from build123d import *

# Parameters (mm, degrees)
SKETCH1_R      = 2.35
EXTRUDE1_DEPTH = 3.1


with BuildPart() as part:
    # Sketch1 → Extrude1 (new body)
    with BuildSketch(Plane.XY):
        Polygon((-33.263157114, 29.408489293), (-41.013157114, 29.408489293), (-41.013157114, 12.158489293), (-33.263157114, 12.158489293), (-33.263157114, 9.058489293), (-18.263157114, 9.058489293), (-18.263157114, 12.158489293), (-10.513157114, 12.158489293), (-10.513157114, 29.408489293), (-18.263157114, 29.408489293), (-18.263157114, 32.508489293), (-33.263157114, 32.508489293), align=None)
        with Locations(Location((-14.388157114, 26.058489293, 0), (0, 0, 180))):
            Circle(SKETCH1_R, mode=Mode.SUBTRACT)
        with Locations(Location((-37.138157114, 26.058489293, 0), (0, 0, 180))):
            Circle(SKETCH1_R, mode=Mode.SUBTRACT)
        with Locations(Location((-25.763157114, 15.508489293, 0), (0, 0, 180))):
            Circle(SKETCH1_R, mode=Mode.SUBTRACT)
        with BuildLine():
            Line((-37.138157114, 21.287155622), (-37.138157114, 14.158489293))
            ThreePointArc((-37.138157114, 14.158489293), (-36.845263895, 13.451382512), (-36.138157114, 13.158489293))
            Line((-36.138157114, 13.158489293), (-33.725119975, 13.158489293))
            ThreePointArc((-33.725119975, 13.158489293), (-33.328320215, 13.240584097), (-32.996670851, 13.473389392))
            Line((-32.996670851, 13.473389392), (-28.585897467, 18.16325141))
            ThreePointArc((-28.585897467, 18.16325141), (-25.763157114, 19.383489293), (-22.940416761, 18.16325141))
            Line((-22.940416761, 18.16325141), (-18.529643377, 13.473389392))
            ThreePointArc((-18.529643377, 13.473389392), (-18.197994013, 13.240584097), (-17.801194253, 13.158489293))
            Line((-17.801194253, 13.158489293), (-15.388157114, 13.158489293))
            ThreePointArc((-15.388157114, 13.158489293), (-14.681050333, 13.451382512), (-14.388157114, 14.158489293))
            Line((-14.388157114, 14.158489293), (-14.388157114, 21.287155622))
            ThreePointArc((-14.388157114, 21.287155622), (-14.611907088, 21.917580794), (-15.183028909, 22.265890734))
            ThreePointArc((-15.183028909, 22.265890734), (-17.128195891, 23.318450516), (-18.180755673, 25.263617499))
            ThreePointArc((-18.180755673, 25.263617499), (-18.529065613, 25.834739319), (-19.159490785, 26.058489293))
            Line((-19.159490785, 26.058489293), (-32.366823443, 26.058489293))
            ThreePointArc((-32.366823443, 26.058489293), (-32.997248615, 25.834739319), (-33.345558555, 25.263617499))
            ThreePointArc((-33.345558555, 25.263617499), (-34.398118337, 23.318450516), (-36.343285319, 22.265890734))
            ThreePointArc((-36.343285319, 22.265890734), (-36.91440714, 21.917580794), (-37.138157114, 21.287155622))
        make_face(mode=Mode.SUBTRACT)
    extrude(amount=EXTRUDE1_DEPTH)


solid = part.part
Here's how the part is built. I have some questions about the finished solid (model axes, mm). A direction names the side the tool comes from. Coordinates: 2 decimals unless noted, no trailing zeros. Loops run counter-clockwise (first coordinate to the right, second up) from the corner with the lowest first, then second, coordinate; pieces in that order, holes last.
1. If we mould it in two halves opening along Y, with no side actions, what happens to faces 1 (the flat face through (-37, 12.158, 2)), 2 (the flat face through (-33.263, 11, 2)), 3 (the flat face through (-17, 13.158, 2))? For each: pulls with the +Y half, pulls with the -Y half, needs draft (parallel to the pull), parting line crosses it, or undercut.
2. I need wall thicknesses on L1, parallel to X at y = 18, z = 0.25; L2, parallel to X at y = 17, z = 1.45; L3, parallel to X at y = 16, z = 1.6. Which ranges of each line are inside material? Lowest first, please.
3. For faces 4 (the flat face through (-33.263, 31, 2)), 5 (the flat face through (-18.263, 31, 2)), 6 (the flat face through (-20.766, 15.851, 1.528)), which set-ups out of +Z, -Z, +X, -X, +Y, -Y let a thin tool reach every point of the face, with its end or its side?
4. Imagine slicing it at C-C, the plane y = 17. Please give me the cut outline in (x, z), and give its area (3 significant figures).
5. Imagine slicing it at A-A, the plane y = 19.75. Please give me the cut outline in (x, z), and give its area (3 significant figures).
6. For P1, Ø1.6, axis at x = -15.5, z = 1, coming from the +Y side; P2, Ø0.9, axis at x = -38, z = 2.5, coming from the -Y side; P3, Ø1.5, axis at y = 30.5, z = 1.5, coming from the -X side, each with a flat end and sliding along its axis, tell me the tip position at first contact or that it passes through.
7. Imagine slicing it at B-B, the plane x = -30. Please give me the cut outline in (y, z).
8. Imagine slicing it at D-D, the plane z = 1.8. Count the separate pieces of the cut face and the enclosed holes in it, and give its area (3 significant figures).
Taken from the geometry:
1. face 1: pulls with the -Y half
1. face 2: needs draft
1. face 3: undercut
2. L1: x = -41.01 to -37.14, -28.74 to -22.79, -14.39 to -10.51
2. L2: x = -41.01 to -37.14, -29.68 to -27.58, -23.95 to -21.85, -14.39 to -10.51
2. L3: x = -41.01 to -37.14, -30.62 to -28.06, -23.47 to -20.91, -14.39 to -10.51
3. face 4: +Z, -Z, -X, +Y
3. face 5: +Z, -Z, +X, +Y
3. face 6: +Z, -Z
4. outline: (-41.01, 0) - (-37.14, 0) - (-37.14, 3.1) - (-41.01, 3.1) - close; (-29.68, 0) - (-27.58, 0) - (-27.58, 3.1) - (-29.68, 3.1) - close; (-23.95, 0) - (-21.85, 0) - (-21.85, 3.1) - (-23.95, 3.1) - close; (-14.39, 0) - (-10.51, 0) - (-10.51, 3.1) - (-14.39, 3.1) - close
4. area: 37.0 mm2
5. outline: (-41.01, 0) - (-37.14, 0) - (-37.14, 3.1) - (-41.01, 3.1) - close; (-14.39, 0) - (-10.51, 0) - (-10.51, 3.1) - (-14.39, 3.1) - close
5. area: 24.0 mm2
6. P1: stops at y = 29.41
6. P2: stops at y = 12.16
6. P3: stops at x = -33.26
7. outline: (9.06, 0) - (16.66, 0) - (16.66, 3.1) - (9.06, 3.1) - close; (26.06, 0) - (32.51, 0) - (32.51, 3.1) - (26.06, 3.1) - close
8. separate pieces: 1
8. enclosed holes: 4
8. area: 355 mm2
